Geometry check sheet. Reference: the model listing, model coordinates, mm. Face numbers are marked on the shaded views. Coordinates: 2 decimals unless noted, no trailing zeros. Order: outer loops, then holes, each group sorted by start corner. A loop starts at its lowest first (then second) coordinate and runs counter-clockwise, first axis right, second up. Notation, with made-up numbers: (-2.75, 7.5) - (30.25, 7.5) arc R25 cw to (30.25, 19.5) - close; hole circle Ø2 at (34.5, 49). An arc over 180 degrees is marked (long way). Use CSV: the item, a comma, the result in double quotes. Start each with the question number.
1) Sectioned sample at B-B, the plane z = 0. Record the cut outline in (x, y) (1 decimal), and give its area (3 significant figures).
2) Thickness scan on probe 1 along Y at (x, z) = (1.5, 0); probe 2 along Z at (x, y) = (0, -3); probe 3 along Z at (x, y) = (1.25, -1). Record the ranges inside material, lowest first. Write a range as [from, to].
3) Sectioned sample at A-A, the plane y = 0. Record the cut outline in (x, z) (3 decimals).
4) Draft check along X on the marked faces 1, 2, 3 and 4. Enter one of: released by +X, released by -X, zero draft, split by the parting line, or undercut.
5) Sectioned sample at C-C, the plane x = 0.25. Record the cut outline in (y, z).
6) Sectioned sample at D-D, the plane x = 1.25. Record the cut outline in (y, z).
7) Depth check by flat-ended pin: P1, Ø1, axis at x = 3, y = -2, coming from the +Z side. Enter the tip coordinate at first touch or a pass-through.
from build123d import *

# Parameters (mm, degrees)
SKETCH1_R                    = 3.556
BOSS_EXTRUDE1_DEPTH          = 3.556
F_30_0_1285_DIAMETER_HOLE1_D = 3.2639
CHAMFER2_SIZE                = 0.381
F_65_0_035_DIAMETER_HOLE2_D  = 0.889


with BuildPart() as part:
    # Sketch1 → Boss-Extrude1 (new, symmetric)
    with BuildSketch(Plane(origin=(0, 0, 0), x_dir=(0, 0, -1), z_dir=(1, 0, 0))):
        Circle(SKETCH1_R)
    extrude(amount=BOSS_EXTRUDE1_DEPTH, both=True)

    # #30 (0.1285) Diameter Hole1 (through all)
    with Locations(Plane(origin=(3.556, 0, 0), x_dir=(0, 0, -1), z_dir=(1, 0, 0))):
        with Locations((0, 0)):
            Hole(F_30_0_1285_DIAMETER_HOLE1_D / 2)

    # Chamfer2
    chamfer2_edges = [part.edges().sort_by_distance(p)[0] for p in [
        (-3.556, 0, 3.556),
        (3.556, 0, 3.556),
    ]]
    chamfer(chamfer2_edges, length=CHAMFER2_SIZE)

    # #65 (0.035) Diameter Hole2 (through all)
    with Locations(Plane(origin=(0, 3.556, 0), x_dir=(1, 0, 0), z_dir=(0, 1, 0))):
        with Locations((0, 0)):
            Hole(F_65_0_035_DIAMETER_HOLE2_D / 2)


solid = part.part
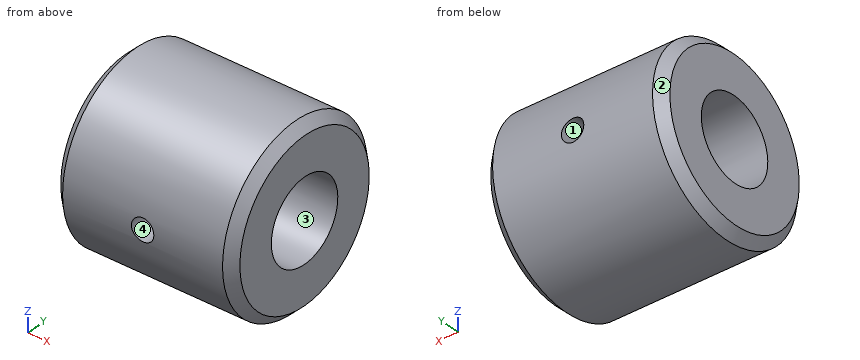
Evaluation:
1,outline,"(-3.6, -3.2) - (-3.2, -3.6) - (-0.4, -3.6) - (-0.4, -1.6) - (-3.6, -1.6) - close; (-3.6, 1.6) - (-0.4, 1.6) - (-0.4, 3.6) - (-3.2, 3.6) - (-3.6, 3.2) - close; (0.4, -3.6) - (3.2, -3.6) - (3.6, -3.2) - (3.6, -1.6) - (0.4, -1.6) - close; (0.4, 1.6) - (3.6, 1.6) - (3.6, 3.2) - (3.2, 3.6) - (0.4, 3.6) - close"
1,area,"23.7 mm²"
2,probe 1,"[-3.56, -1.63], [1.63, 3.56]"
2,probe 2,"[-1.91, -0.44], [0.44, 1.91]"
2,probe 3,"[-3.41, -1.29], [1.29, 3.41]"
3,outline,"(-3.556, -3.175) - (-3.175, -3.556) - (3.175, -3.556) - (3.556, -3.175) - (3.556, -1.632) - (-3.556, -1.632) - close; (-3.556, 1.632) - (3.556, 1.632) - (3.556, 3.175) - (3.175, 3.556) - (-3.175, 3.556) - (-3.556, 3.175) - close"
4,face 1,"undercut"
4,face 2,"released by -X"
4,face 3,"zero draft"
4,face 4,"undercut"
5,outline,"(-3.54, -0.37) arc R3.56 ccw to (3.54, -0.37) - (1.59, -0.37) arc R1.63 cw to (-1.59, -0.37) - close; (-3.54, 0.37) - (-1.59, 0.37) arc R1.63 cw to (1.59, 0.37) - (3.54, 0.37) arc R3.56 ccw to start"
6,outline,"circle Ø7.11 at (0, 0); hole circle Ø3.26 at (0, 0)"
7,P1,"z = 3.22"
